Build history of the part. All positions in model axes, mm. A direction names the side the tool comes from. Round coordinates to 2 decimals unless told otherwise and drop trailing zeros. Order: outer loops, then holes, each group sorted by start corner. A loop starts at its lowest first (then second) coordinate and runs counter-clockwise, first axis right, second up. Notation, with made-up numbers: (-8, 45.5) -> (51, 45.5) arc R13 cw to (51, 56.5) -> close; hole circle Ø11 at (-10, 7). An arc over 180 degrees is marked (long way). Write item = value, one per line.
from build123d import *

# Parameters (mm, degrees)
SKETCH1_W             = 17
SKETCH1_H             = 25
BOSS_EXTRUDE1_DEPTH   = 3
BOSS_EXTRUDE1_2_DEPTH = 3
SKETCH2_W             = 86
SKETCH2_H             = 12
BOSS_EXTRUDE2_DEPTH   = 3
SKETCH3_R             = 1.3
CUT_EXTRUDE1_DEPTH    = 3
SKETCH4_R             = 1.44
CUT_EXTRUDE2_DEPTH    = 3
BOSS_EXTRUDE3_START   = 18
BOSS_EXTRUDE3_DEPTH   = 3
BOSS_EXTRUDE4_START   = -18
BOSS_EXTRUDE4_DEPTH   = 3
FILLET1_R             = 2
FILLET2_R             = 4


with BuildPart() as part:
    # Sketch1 → Boss-Extrude1 (new body)
    with BuildSketch(Plane(origin=(0, 0, 0), x_dir=(1, 0, 0), z_dir=(0, 1, 0))):
        with Locations((-26.5, 16)):
            Rectangle(SKETCH1_W, SKETCH1_H)
    extrude(amount=BOSS_EXTRUDE1_DEPTH)


with BuildPart() as body_2:
    # Sketch1 → Boss-Extrude1 2 (new body)
    with BuildSketch(Plane(origin=(0, 0, 0), x_dir=(1, 0, 0), z_dir=(0, 1, 0))):
        with Locations((26.5, 16)):
            Rectangle(SKETCH1_W, SKETCH1_H)
    extrude(amount=BOSS_EXTRUDE1_2_DEPTH)


with BuildPart() as body_3:
    # Sketch2 → Boss-Extrude2 (new body)
    with BuildSketch(Plane(origin=(0, 0, 0), x_dir=(1, 0, 0), z_dir=(0, 0.2588190451025247, -0.9659258262890672))):
        with Locations((0, -20)):
            Rectangle(SKETCH2_W, SKETCH2_H)
    extrude(amount=BOSS_EXTRUDE2_DEPTH)

    # Sketch4 → Cut-Extrude2 (cut)
    with BuildSketch(Plane(origin=(0, 0, 0), x_dir=(1, 0, 0), z_dir=(0, -0.25881904510252474, 0.9659258262890673))):
        with Locations(Location((-37.35, 20, 0), (0, 0, 270))):
            Circle(SKETCH4_R)
        with Locations(Location((37.35, 20, 0), (0, 0, 270))):
            Circle(SKETCH4_R)
    extrude(amount=-CUT_EXTRUDE2_DEPTH, mode=Mode.SUBTRACT)


with BuildPart() as cut_extrude1_tool:
    # Sketch3 → Cut-Extrude1 (new body)
    with BuildSketch(Plane.XZ):
        with Locations(Location((30, -25, 0), (0, 0, 270))):
            Circle(SKETCH3_R)
        with Locations(Location((30, -7, 0), (0, 0, 270))):
            Circle(SKETCH3_R)
        with Locations(Location((-30, -25, 0), (0, 0, 270))):
            Circle(SKETCH3_R)
        with Locations(Location((-30, -7, 0), (0, 0, 270))):
            Circle(SKETCH3_R)
    extrude(amount=-CUT_EXTRUDE1_DEPTH)


with BuildPart() as part_1:
    add(part.part)

    # Cut-Extrude1: cut by cut_extrude1_tool
    add(cut_extrude1_tool.part, mode=Mode.SUBTRACT)



with BuildPart() as body_2_1:
    add(body_2.part)

    # Cut-Extrude1: cut by cut_extrude1_tool
    add(cut_extrude1_tool.part, mode=Mode.SUBTRACT)


    add(body_3.part)  # Boss-Extrude3 merges body 3
    # Sketch5 → Boss-Extrude3 (add)
    with BuildSketch(Plane(origin=(0, 0, 0), x_dir=(0, 0, -1), z_dir=(1, 0, 0)).offset(BOSS_EXTRUDE3_START)):
        Polygon((3.5, 3), (28.5, 3), (28.5, 4.5), (-2.382628954, 26.278757186), (-3.831517694, 25.890528619), (-0.725689153, 14.299418703), (-2.174577892, 13.911190136), (3.5, 1.5), align=None)
    extrude(amount=BOSS_EXTRUDE3_DEPTH)


with BuildPart() as part_2:
    add(part_1.part)

    add(body_2_1.part)  # Boss-Extrude4 merges body 2
    # Sketch5<2> → Boss-Extrude4 (add)
    with BuildSketch(Plane(origin=(0, 0, 0), x_dir=(0, 0, -1), z_dir=(1, 0, 0)).offset(BOSS_EXTRUDE4_START)):
        Polygon((3.5, 3), (28.5, 3), (28.5, 4.5), (-2.382628954, 26.278757186), (-3.831517694, 25.890528619), (-0.725689153, 14.299418703), (-2.174577892, 13.911190136), (3.5, 1.5), align=None)
    extrude(amount=-BOSS_EXTRUDE4_DEPTH)

    # Fillet1
    # the kernel refuses this fillet: 2 mm, written as the material it adds along each edge
    with BuildSketch(Plane(origin=(-21, 3, -3.5), x_dir=(0, 1, 0), z_dir=(0, 0, -1))) as fillet1_piece_1_section:
        with BuildLine():
            CenterArc((FILLET1_R, -FILLET1_R), FILLET1_R, 90, 90)
            Line((0, -FILLET1_R), (0, 0))
            Line((0, 0), (FILLET1_R, 0))
        make_face()
    fillet1_piece_1 = extrude(amount=25, mode=Mode.PRIVATE)
    fillet1_piece_1 = split(fillet1_piece_1, bisect_by=Plane(origin=(-21.452953813, 10.041317551, -20.642322338), z_dir=(0, -0.8172264215847361, 0.5763167322434836)), keep=Keep.TOP, mode=Mode.PRIVATE)
    add(fillet1_piece_1)
    with BuildSketch(Plane(origin=(21, 3, -3.5), x_dir=(0, 1, 0), z_dir=(0, 0, -1))) as fillet1_piece_2_section:
        with BuildLine():
            CenterArc((FILLET1_R, FILLET1_R), FILLET1_R, 180, 90)
            Line((0, FILLET1_R), (0, 0))
            Line((0, 0), (FILLET1_R, 0))
        make_face()
    fillet1_piece_2 = extrude(amount=25, mode=Mode.PRIVATE)
    fillet1_piece_2 = split(fillet1_piece_2, bisect_by=Plane(origin=(21.452953813, 10.041317551, -20.642322338), z_dir=(0, -0.8172264215847361, 0.5763167322434836)), keep=Keep.TOP, mode=Mode.PRIVATE)
    add(fillet1_piece_2)
    with BuildSketch(Plane(origin=(-18, 25.890528619, 3.831517694), x_dir=(1, 0, 0), z_dir=(0, -0.9659258262890673, -0.2588190451025247))) as fillet1_piece_3_section:
        with BuildLine():
            CenterArc((FILLET1_R, -FILLET1_R), FILLET1_R, 90, 90)
            Line((0, -FILLET1_R), (0, 0))
            Line((0, 0), (FILLET1_R, 0))
        make_face()
    fillet1_piece_3 = extrude(amount=12, mode=Mode.PRIVATE)
    fillet1_piece_3 = split(fillet1_piece_3, bisect_by=Plane(origin=(-17.546921316, 24.007524822, -0.83801517), z_dir=(0, -0.8172264215847361, 0.5763167322434836)), keep=Keep.TOP, mode=Mode.PRIVATE)
    add(fillet1_piece_3)
    with BuildSketch(Plane(origin=(-21, 25.890528619, 3.831517694), x_dir=(0, 0.2588190451025247, -0.9659258262890672), z_dir=(0, -0.9659258262890673, -0.2588190451025247))) as fillet1_piece_4_section:
        with BuildLine():
            CenterArc((FILLET1_R, -FILLET1_R), FILLET1_R, 90, 90)
            Line((0, -FILLET1_R), (0, 0))
            Line((0, 0), (FILLET1_R, 0))
        make_face()
    fillet1_piece_4 = extrude(amount=12, mode=Mode.PRIVATE)
    fillet1_piece_4 = split(fillet1_piece_4, bisect_by=Plane(origin=(-21.453078684, 24.007524822, -0.838015171), z_dir=(0, -0.8172264215847361, 0.5763167322434836)), keep=Keep.TOP, mode=Mode.PRIVATE)
    add(fillet1_piece_4)
    with BuildSketch(Plane(origin=(21, 25.890528619, 3.831517694), x_dir=(1, 0, 0), z_dir=(0, -0.9659258262890673, -0.2588190451025247))) as fillet1_piece_5_section:
        with BuildLine():
            CenterArc((FILLET1_R, -FILLET1_R), FILLET1_R, 90, 90)
            Line((0, -FILLET1_R), (0, 0))
            Line((0, 0), (FILLET1_R, 0))
        make_face()
    fillet1_piece_5 = extrude(amount=12, mode=Mode.PRIVATE)
    fillet1_piece_5 = split(fillet1_piece_5, bisect_by=Plane(origin=(21.453078684, 24.007524822, -0.83801517), z_dir=(0, -0.8172264215847361, 0.5763167322434836)), keep=Keep.TOP, mode=Mode.PRIVATE)
    add(fillet1_piece_5)
    with BuildSketch(Plane(origin=(18, 25.890528619, 3.831517694), x_dir=(-1.776356839400251e-15, 0.25881904510252474, -0.9659258262890673), z_dir=(0, -0.9659258262890673, -0.2588190451025247))) as fillet1_piece_6_section:
        with BuildLine():
            CenterArc((FILLET1_R, -FILLET1_R), FILLET1_R, 90, 90)
            Line((0, -FILLET1_R), (0, 0))
            Line((0, 0), (FILLET1_R, 0))
        make_face()
    fillet1_piece_6 = extrude(amount=12, mode=Mode.PRIVATE)
    fillet1_piece_6 = split(fillet1_piece_6, bisect_by=Plane(origin=(17.546921316, 24.007524822, -0.838015171), z_dir=(0, -0.8172264215847361, 0.5763167322434836)), keep=Keep.TOP, mode=Mode.PRIVATE)
    add(fillet1_piece_6)

    # Fillet2
    fillet2_edges = [part_2.edges().sort_by_distance(p)[0] for p in [
        (43, 13.911190136, 2.174577892),
        (-43, 13.911190136, 2.174577892),
        (-43, 25.502300051, 5.280406433),
        (43, 25.502300051, 5.280406433),
        (35, 1.5, -28.5),
        (35, 1.5, -3.5),
        (-35, 1.5, -28.5),
        (-35, 1.5, -3.5),
    ]]
    fillet(fillet2_edges, radius=FILLET2_R)


solid = part_2.part
Q1. Cut at B-B, the plane y = 10. List the corners of the cut face in (x, z), and give its area (3 significant figures).
Check values:
outline = (-21, -20.7) -> (-18, -20.7) -> (-18, 0.39) -> (-21, 0.39) -> close; (18, -20.7) -> (21, -20.7) -> (21, 0.39) -> (18, 0.39) -> close
area = 127 mm²
Q2. Mould opens along Y. For faces 1 (the face through (-33.14, 20.014, 2.257)), 2 (the face through (19.479, 7.792, -0.623)), 3 (the face through (30.39, 1.48, -8.24)), 4 (the face through (-35.922, 19.882, 3.796)) say: released by +Y, released by -Y, zero draft, split by the parting line, or undercut.
Check values:
face_1 = released by +Y
face_2 = released by -Y
face_3 = zero draft
face_4 = undercut
Q3. Flat gauge pins, fed straight in: pin 1 (2.5 mm diameter, centred on x = -30, z = -25, fed in from +Y); pin 2 (9.5 mm diameter, centred on x = -30.5, z = -16.5, fed in from +Y); pin 3 (3 mm diameter, centred on y = 10, z = -0.5, fed in from -X); pin 4 (1.5 mm diameter, centred on y = 1.5, z = -14, fed in from -X). Where does each tip first touch, or does it go through?
Check values:
pin_1 = through
pin_2 = 3
pin_3 = -21
pin_4 = -35
Q4. Cut at C-C, the plane z = -9.5. List the corners of the cut face in (x, y), and give its area (3 significant figures).
Check values:
outline = (-35, 0) -> (-18, 0) -> (-18, 17.9) -> (-21, 17.9) -> (-21, 5) arc R2 cw to (-23, 3) -> (-35, 3) -> close; (18, 0) -> (35, 0) -> (35, 3) -> (23, 3) arc R2 cw to (21, 5) -> (21, 17.9) -> (18, 17.9) -> close
area = 193 mm²
Q5. Probe probe 1 along X at (y, z) = (21.75, -0.5); probe 2 along X at (y, z) = (0.7, -7); probe 3 along X at (y, z) = (4.5, -17). List the from-to ranges inside material, lowest first.
Check values:
probe_1 = -21 to -18, 18 to 21
probe_2 = -34.97 to -31.3, -28.7 to -18, 18 to 28.7, 31.3 to 34.97
probe_3 = -21.06 to -18, 18 to 21.06
Q6. Which spindle directions (+Z, -Z, +X, -X, +Y, -Y) get a long thin tool onto all of the face, cutting with end or side? Do faces 5 (the face through (-0.224, 20.014, 2.257)), 6 (the face through (-29, 3, -16)), 7 (the face through (32.86, 20.014, 2.257)). Say none if no direction does.
Check values:
face_5 = -Z, +Y
face_6 = +Z, -Z, -X, +Y
face_7 = -Z, +X, +Y
Q7. Cut at A-A, the plane x = -27. List the corners of the cut face in (y, z), and give its area (3 significant figures).
Check values:
outline = (0, -28.5) -> (3, -28.5) -> (3, -3.5) -> (0, -3.5) -> close; (13.52, 3.62) -> (14.3, 0.73) -> (25.89, 3.83) -> (25.11, 6.73) -> close
area = 111 mm²
Q8. Cut at D-D, the plane x = -0.5. List the corners of the cut face in (y, z), and give its area (3 significant figures).
Check values:
outline = (13.52, 3.62) -> (14.3, 0.73) -> (25.89, 3.83) -> (25.11, 6.73) -> close
area = 36.0 mm²
